For this review, take the finished solid that the model builds, in its own axes (mm). A direction names the side the tool comes from. Coordinates: 2 decimals unless noted, no trailing zeros. Write each loop counter-clockwise with the first axis right and the second up, starting at its lowest first coordinate (ties: lowest second). Pieces come first, ordered by that corner, then holes.
1) Insertion check: P1, Ø3, axis at x = 23.5, y = 3, coming from the -Z side; P2, Ø8, axis at x = -21, y = 41.5, coming from the -Z side; P3, Ø6, axis at x = 105.5, y = 34.5, coming from the -Z side. Each pin has a flat end and moves straight along its axis. Give the tip position at first contact, or say it passes through.
2) Mouldability with a two-part tool opening along X and no side actions: class faces 6 (the face through (150, 51, -2)), 7 (the face through (-1, 95, -25)), 8 (the face through (-150, 51, -2)) as pulls with the +X half, pulls with the -X half, needs draft (parallel to the pull), parting line crosses it, or undercut.
3) To check wall thickness, follow line 1 along Z through (x, y) = (-117, 96); line 2 along X through (y, z) = (95, 49); line 3 along Y through (x, z) = (12, 5). State the ranges of each line that lie inside material, in increasing order.
4) For faces 1 (the face through (93.91, 95.07, 24.65)), 2 (the face through (-2, 5, 100)), 3 (the face through (-2, 95, 100)), 4 (the face through (-2, 5, -100)), 5 (the face through (-2, 95, -100)), list the 3-axis set-ups (+Z, -Z, +X, -X, +Y, -Y) from which the entire face can be reached by the end or side of a thin tool; tool diameter is ignored.
5) We need section C-C on y = 19.5. Write out the cut boundary in (x, z), then the cut area to 3 significant figures.
6) We need section D-D on x = 60. Write out the cut boundary in (y, z), then the cut area to 3 significant figures.
7) We need section A-A on x = 15. Write out the cut boundary in (y, z), then the cut area to 3 significant figures.
8) We need section B-B on z = -5. Write out the cut boundary in (x, y), then the cut area to 3 significant figures.
from build123d import *

# Parameters (mm, degrees)
SKETCH1_W           = 300
SKETCH1_H           = 200
BOSS_EXTRUDE2_DEPTH = 100
SKETCH2_R           = 40
BOSS_EXTRUDE3_DEPTH = 300
CUT_EXTRUDE1_DEPTH  = 10


with BuildPart() as part:
    # Sketch1 → Boss-Extrude2 (new body)
    with BuildSketch(Plane(origin=(0, 0, 0), x_dir=(1, 0, 0), z_dir=(0, 1, 0))):
        Rectangle(SKETCH1_W, SKETCH1_H)
    extrude(amount=BOSS_EXTRUDE2_DEPTH)

    # Sketch2 → Boss-Extrude3 (add)
    with BuildSketch(Plane.ZY.offset(150)):
        with Locations((100, 50)):
            Circle(SKETCH2_R)
        with Locations((-100, 50)):
            Circle(SKETCH2_R)
    extrude(amount=-BOSS_EXTRUDE3_DEPTH)

    # Sketch3 → Cut-Extrude1 (cut)
    with BuildSketch(Plane(origin=(0, 100, 0), x_dir=(1, 0, 0), z_dir=(0, 1, 0))):
        Polygon((50, 25), (50, 50), (136.602540378, 0), (50, -50), (50, -25), (-50, -25), (-50, 25), align=None)
    extrude(amount=-CUT_EXTRUDE1_DEPTH, mode=Mode.SUBTRACT)


solid = part.part
Result:
1. P1: stops at z = -100
1. P2: stops at z = -139.75
1. P3: stops at z = -138
2. face 6: pulls with the +X half
2. face 7: undercut
2. face 8: pulls with the -X half
3. line 1: z = -100 to 100
3. line 2: x = -150 to 50, 51.73 to 150
3. line 3: y = 0 to 90
4. face 1: +Y
4. face 2: +Z, +X, -X, -Y
4. face 3: +Z, +X, -X, +Y
4. face 4: -Z, +X, -X, -Y
4. face 5: -Z, +X, -X, +Y
5. outline: (-150, -125.88) - (150, -125.88) - (150, 125.88) - (-150, 125.88) - close
5. area: 75,500 mm2
6. outline: (0, -100) - (10, -100) arc R40 ccw to (90, -100) - (100, -100) - (100, -44.23) - (90, -44.23) - (90, 44.23) - (100, 44.23) - (100, 100) - (90, 100) arc R40 ccw to (10, 100) - (0, 100) - close
6. area: 24,100 mm2
7. outline: (0, -100) - (10, -100) arc R40 ccw to (90, -100) - (100, -100) - (100, -25) - (90, -25) - (90, 25) - (100, 25) - (100, 100) - (90, 100) arc R40 ccw to (10, 100) - (0, 100) - close
7. area: 24,500 mm2
8. outline: (-150, 0) - (150, 0) - (150, 100) - (127.94, 100) - (127.94, 90) - (-50, 90) - (-50, 100) - (-150, 100) - close
8. area: 28,200 mm2
